from build123d import *

# Parameters (mm, degrees)
F0_W     = 100
F0_H     = 100
F1_DEPTH = 4.5
F2_W     = 100
F2_H     = 100
F2_W_2   = 91
F2_H_2   = 91
F3_DEPTH = 15
F4_W     = 100
F4_H     = 100
F5_DEPTH = 4.5
F7_DEPTH = 6


with BuildPart() as f1:
    # F0 (on Top) → F1 (new body)
    with BuildSketch(Plane.XY):
        Rectangle(F0_W, F0_H)
    extrude(amount=F1_DEPTH)

    # F2 (on face) → F3 (join)
    with BuildSketch(Plane.XY.offset(4.5)):
        Rectangle(F2_W, F2_H)
        Rectangle(F2_W_2, F2_H_2, mode=Mode.SUBTRACT)
    extrude(amount=F3_DEPTH)

    # F4 (on face) → F5 (join)
    with BuildSketch(Plane.XY.offset(19.5)):
        Rectangle(F4_W, F4_H)
    extrude(amount=F5_DEPTH)

    # F6 (on face) → F7 (cut)
    with BuildSketch(Plane.XY.offset(24)):
        Polygon((44.2315, -2.125047), (44.2315, 6.574953), (18.081121, 6.574953), (18.081121, 32.144), (-5.230078, 32.144), (-5.230078, -21.518026), (-27.644688, -21.518026), (-27.644688, 15.241936), (-44.2315, 15.241936), (-44.2315, 6.541936), (-35.896394, 6.541936), (-35.896394, -32.144), (3.918216, -32.144), (3.918216, 23.444234), (9.829416, 23.444234), (9.829416, -4.051022), (44.2315, -4.051022), align=None)
    extrude(amount=-F7_DEPTH, mode=Mode.SUBTRACT)


solid = f1.part
Work out the finished part from the listing and answer in its coordinate system (mm). A direction names the side the tool comes from. Coordinates: 2 decimals unless noted, no trailing zeros. Write each loop counter-clockwise with the first axis right and the second up, starting at its lowest first coordinate (ties: lowest second). Pieces come first, ordered by that corner, then holes.
1. The part is cut by section A-A, the plane x = -41. Write down the section's boundary in (y, z), and give its area (3 significant figures).
Results list:
outline: (-50, 0) - (50, 0) - (50, 24) - (15.24, 24) - (15.24, 19.5) - (45.5, 19.5) - (45.5, 4.5) - (-45.5, 4.5) - (-45.5, 19.5) - (6.54, 19.5) - (6.54, 24) - (-50, 24) - close
area: 996 mm2
2. For faces 1 (the flat face through (-50, -1, 12)), 2 (the flat face through (-27.645, -3, 22)), 3 (the flat face through (-1, 1, 4.5)), determine the directions among +Z, -Z, +X, -X, +Y, -Y from which every point of the face is accessible in a straight line to the end or side of a thin tool.
Results list:
face 1: +Z, -Z, -X, +Y, -Y
face 2: +Z
face 3: none
3. For a pull along Z with two mould halves and no side action, classify faces 4 (the flat face through (-35.896, -13, 22)), 5 (the flat face through (9, 1, 19.5)), 6 (the flat face through (-1, 1, 0)) as +Z half, -Z half, draft (parallel to the pull), parting line (faces both ways), or undercut.
Results list:
face 4: draft
face 5: undercut
face 6: -Z half
4. The part is cut by section B-B, the plane z = 12.75. Write down the section's boundary in (x, y).
Results list:
outline: (-50, -50) - (50, -50) - (50, 50) - (-50, 50) - close; hole (-45.5, -45.5) - (45.5, -45.5) - (45.5, 45.5) - (-45.5, 45.5) - close
5. Consider line 1 along X through (y, z) = (-8, 21.25); line 2 along Y through (x, z) = (-40.5, 16.5). Determine where each line is inside the solid, lowest interval first.
Results list:
line 1: x = -50 to -35.9, -27.64 to -5.23, 3.92 to 50
line 2: y = -50 to -45.5, 45.5 to 50
6. The part is cut by section C-C, the plane y = -8.5. Write down the section's boundary in (x, z).
Results list:
outline: (-50, 0) - (50, 0) - (50, 24) - (3.92, 24) - (3.92, 19.5) - (45.5, 19.5) - (45.5, 4.5) - (-45.5, 4.5) - (-45.5, 19.5) - (-35.9, 19.5) - (-35.9, 24) - (-50, 24) - close; (-27.64, 19.5) - (-5.23, 19.5) - (-5.23, 24) - (-27.64, 24) - close
7. The part is cut by section D-D, the plane y = 36.5. Write down the section's boundary in (x, z), and give its area (4 significant figures).
Results list:
outline: (-50, 0) - (50, 0) - (50, 24) - (-50, 24) - close; hole (-45.5, 4.5) - (45.5, 4.5) - (45.5, 19.5) - (-45.5, 19.5) - close
area: 1,035 mm2
8. A flat-ended cylindrical pin translates along its axis: pin 1 (10 mm diameter, centred on x = 22.5, y = 8, fed in from -Z). Find the tip coordinate at first contact, or state that the pin passes through.
Results list:
pin 1: stops at z = 0
